Check sheet for the drawn part. Datum: minimum x, y, z corner. Units: mm. A direction names the side the tool comes from. Give positions to 0.01 mm unless a question says otherwise; leave off trailing zeros. Write each loop counter-clockwise with the first axis right and the second up, starting at its lowest first coordinate (ties: lowest second). Pieces come first, ordered by that corner, then holes.
(1) Depth check by flat-ended pin: P1, Ø4, axis at x = 7, y = 39.5, coming from the -Z side; P2, Ø4.5, axis at y = 16.25, z = 10.58, coming from the +X side. Enter the tip coordinate at first touch or a pass-through.
(2) Tool access check on the marked faces 1 and 2. Record the directions out of +Z, -Z, +X, -X, +Y, -Y that give a thin tool (end or side, any length) a straight path to the whole face; none if there is none.
(3) Thickness scan on line 1 along Y through (x, z) = (37, 47.7); line 2 along Y through (x, z) = (2, 24); line 3 along Y through (x, z) = (17, 44). Record the ranges inside material, lowest first.
(4) Mould release check, pull along Y, two halves, no side actions. Record for the marked faces 3, 4 and 5: +Y half, -Y half, draft (parallel to the pull), parting line (faces both ways), or undercut.
(5) Cross-section at A-A (y = 24). Record the boundary of the cut face in (x, z).
(6) Cross-section at C-C (y = 16.25). Record the boundary of the cut face in (x, z) (1 decimal).
(7) Cross-section at D-D (z = 17). Record the boundary of the cut face in (x, y).
(8) Cross-section at B-B (x = 7). Record the boundary of the cut face in (y, z) (1 decimal).
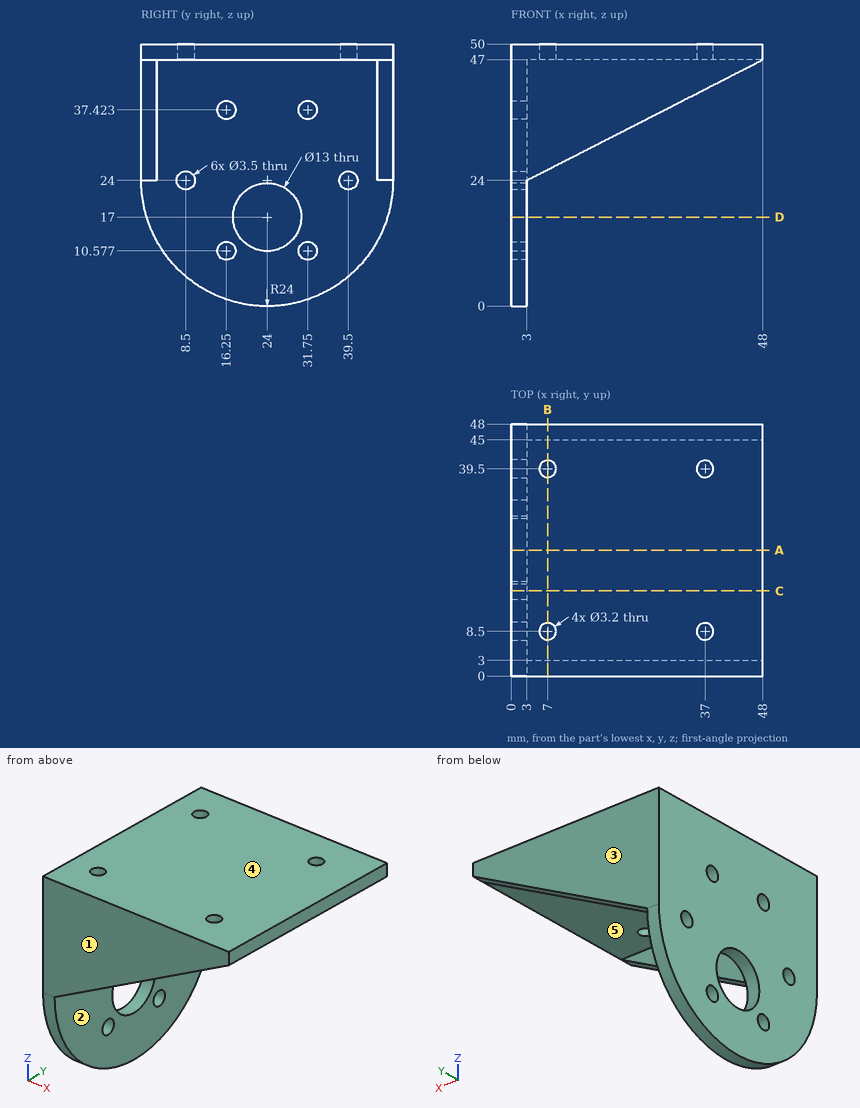
Reply:
1. P1: stops at z = 47
1. P2: stops at x = 3
2. face 1: +Z, -Z, +X, -X, -Y
2. face 2: -Z, +X
3. line 1: y = 0 to 6.9, 10.1 to 37.9, 41.1 to 48
3. line 2: y = 0 to 6.75, 10.25 to 37.75, 41.25 to 48
3. line 3: y = 0 to 3, 45 to 48
4. face 3: +Y half
4. face 4: draft
4. face 5: undercut
5. outline: (0, 0) - (3, 0) - (3, 10.5) - (0, 10.5) - close; (0, 23.5) - (3, 23.5) - (3, 47) - (48, 47) - (48, 50) - (0, 50) - close
6. outline: (0, 1.3) - (3, 1.3) - (3, 8.8) - (0, 8.8) - close; (0, 12.3) - (3, 12.3) - (3, 35.7) - (0, 35.7) - close; (0, 39.2) - (3, 39.2) - (3, 47) - (48, 47) - (48, 50) - (0, 50) - close
7. outline: (0, 1.04) - (3, 1.04) - (3, 17.5) - (0, 17.5) - close; (0, 30.5) - (3, 30.5) - (3, 46.96) - (0, 46.96) - close
8. outline: (0, 26) - (3, 26) - (3, 47) - (6.9, 47) - (6.9, 50) - (0, 50) - close; (10.1, 47) - (37.9, 47) - (37.9, 50) - (10.1, 50) - close; (41.1, 47) - (45, 47) - (45, 26) - (48, 26) - (48, 50) - (41.1, 50) - close
